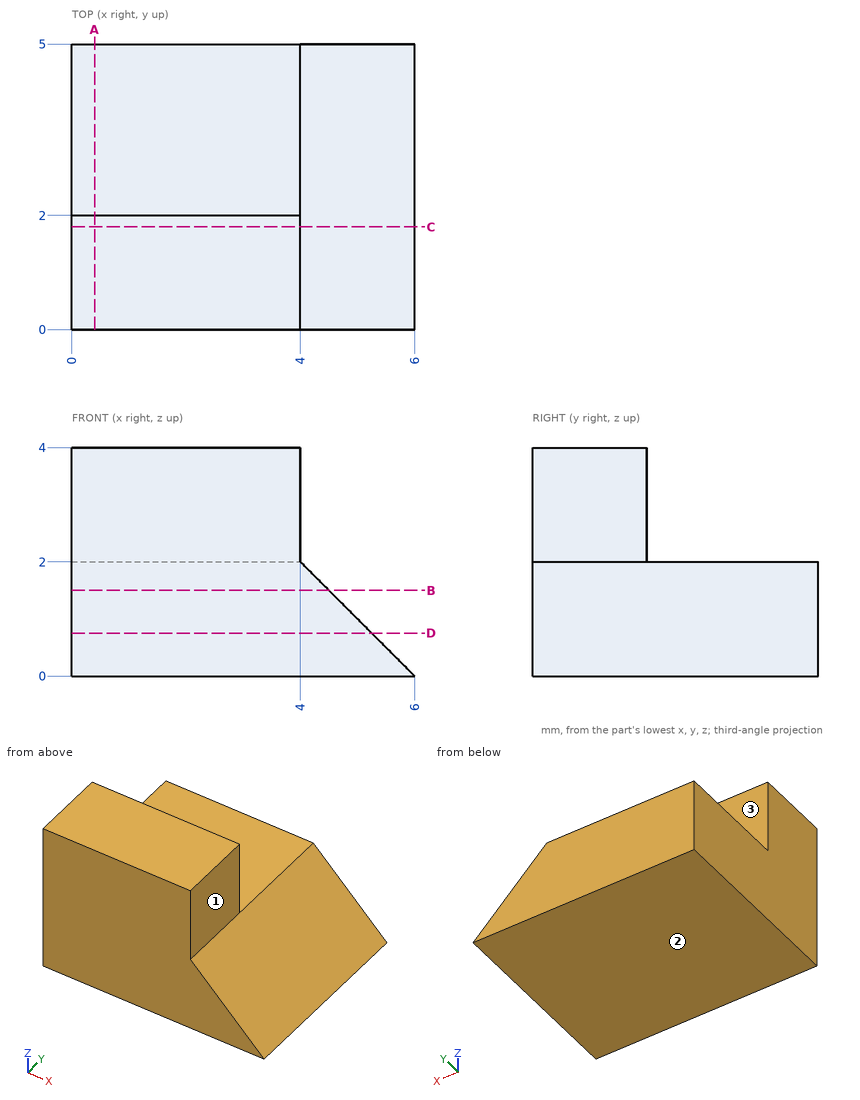
Geometry: see drawing. Coordinates: mm, zero at the bounding-box minimum. A direction names the side the tool comes from. Give positions to 0.01 mm unless a question says otherwise; leave off trailing zeros. Order: outer loops, then holes, each group sorted by start corner. A loop starts at its lowest first (then second) coordinate and runs counter-clockwise, first axis right, second up.
Q1. Section B-B on z = 1.5. Output: boundary loops of the cut face in (x, y), and give its area (3 significant figures).
Checked values:
outline: (0, 0) - (4.5, 0) - (4.5, 5) - (0, 5) - close
area: 22.5 mm2
Q2. Contact query for flat-ended pins moving along their axis: pin 1 Ø2 at (x, z) = (2.5, 3.5) entering from +Y; pin 2 Ø1.5 at (x, y) = (2.5, 4) entering from +Z; pin 3 Ø1.6 at (y, z) = (1.5, 3.5) entering from +X. Output: stop coordinate, or through.
Checked values:
pin 1: stops at y = 2
pin 2: stops at z = 2
pin 3: stops at x = 4
Q3. Set-up query: the marked faces 1, 2 and 3. Return all of +Z, -Z, +X, -X, +Y, -Y with unobstructed straight access to the full face (end or side cutting, diameter ignored); none if empty.
Checked values:
face 1: +Z, +X, +Y, -Y
face 2: -Z, +X, -X, +Y, -Y
face 3: +Z, +X, -X, +Y
Q4. Section D-D on z = 0.75. Output: boundary loops of the cut face in (x, y), and give its area (4 significant figures).
Checked values:
outline: (0, 0) - (5.25, 0) - (5.25, 5) - (0, 5) - close
area: 26.25 mm2
Q5. Section C-C on y = 1.8. Output: boundary loops of the cut face in (x, z), and give its area (3 significant figures).
Checked values:
outline: (0, 0) - (6, 0) - (4, 2) - (4, 4) - (0, 4) - close
area: 18.0 mm2
Q6. Section A-A on x = 0.4. Output: boundary loops of the cut face in (y, z), and give its area (3 significant figures).
Checked values:
outline: (0, 0) - (5, 0) - (5, 2) - (2, 2) - (2, 4) - (0, 4) - close
area: 14.0 mm2
Q7. Ray query, probe 1 along X at (y, z) = (4.3, 1); probe 2 along Y at (x, z) = (0.75, 3.7). Return the intervals inside material, ascending.
Checked values:
probe 1: x = 0 to 5
probe 2: y = 0 to 2
